from build123d import *

# Parameters (mm, degrees)
BOSS_EXTRUDE1_DEPTH = 35
SKETCH2_R           = 0.8
CUT_EXTRUDE1_DEPTH  = 6
SKETCH3_R           = 2.55
CUT_EXTRUDE2_DEPTH  = 6


with BuildPart() as part:
    # Sketch1 → Boss-Extrude1 (new body)
    with BuildSketch(Plane.XY):
        Polygon((-45.495099545, 30), (-5.495099545, 30), (-5.495099545, 0), (0, 0), (0, 35), (-51, 35), (-51, 0), (-45.495099545, 0), align=None)
    extrude(amount=-BOSS_EXTRUDE1_DEPTH)

    # Sketch2 → Cut-Extrude1 (cut)
    with BuildSketch(Plane.ZY.offset(51)):
        with Locations((-13.063320716, 15.474711623)):
            Circle(SKETCH2_R)
        with Locations((-22.063320716, 15.474711623)):
            Circle(SKETCH2_R)
    extrude(amount=-CUT_EXTRUDE1_DEPTH, mode=Mode.SUBTRACT)

    # Sketch3 → Cut-Extrude2 (cut)
    with BuildSketch(Plane(origin=(0, 35, 0), x_dir=(1, 0, 0), z_dir=(0, 1, 0))):
        with Locations(Location((-39, 31.663775096, 0), (0, 0, 180))):
            Circle(SKETCH3_R)
        with Locations(Location((-39, 11.663775096, 0), (0, 0, 180))):
            Circle(SKETCH3_R)
        with Locations(Location((-19.15, 31.663775096, 0), (0, 0, 180))):
            Circle(SKETCH3_R)
        with Locations(Location((-19.15, 11.663775096, 0), (0, 0, 180))):
            Circle(SKETCH3_R)
        with Locations(Location((-29, 21.663775096, 0), (0, 0, 180))):
            Circle(SKETCH3_R)
    extrude(amount=-CUT_EXTRUDE2_DEPTH, mode=Mode.SUBTRACT)


solid = part.part
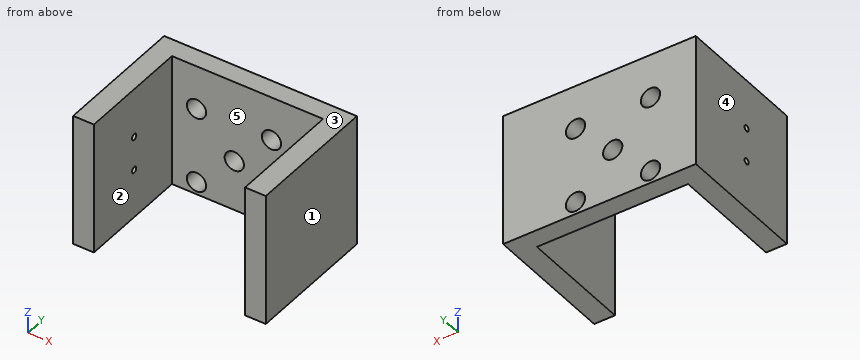
Build history of the part. All positions in model axes, mm. Face numbers are marked on the shaded views. A direction names the side the tool comes from. Round coordinates to 2 decimals unless told otherwise and drop trailing zeros. Write each loop counter-clockwise with the first axis right and the second up, starting at its lowest first coordinate (ties: lowest second). Pieces come first, ordered by that corner, then holes. Notation, with made-up numbers: M -15.75,-0.5 L 37.25,-0.5 A15 ccw 37.25,21.5 Z; hole C -15.5,-12 d10. An arc over 180 degrees is marked long. Answer in a Markdown table with one row per item.
1. Probe L1, parallel to Z at x = -19.15, y = 32.5; L2, parallel to X at y = 12, z = -12.5; L3, parallel to Y at x = -37, z = -14.5. List the from-to ranges inside material, lowest first. Write a range as [from, to].
Geometry check:
| item | result |
|---|---|
| L1 | [-35, -34.21], [-29.11, -14.21], [-9.11, 0] |
| L2 | [-51, -45.5], [-5.5, 0] |
| L3 | [30, 35] |
2. Saw through at B-B (x = -29). List the corners of the cut face in (y, z).
Geometry check:
| item | result |
|---|---|
| outline | M 30,-35 L 35,-35 L 35,-24.21 L 30,-24.21 Z; M 30,-19.11 L 35,-19.11 L 35,0 L 30,0 Z |
3. Saw through at D-D (x = -19.15). List the corners of the cut face in (y, z).
Geometry check:
| item | result |
|---|---|
| outline | M 30,-35 L 35,-35 L 35,-34.21 L 30,-34.21 Z; M 30,-29.11 L 35,-29.11 L 35,-14.21 L 30,-14.21 Z; M 30,-9.11 L 35,-9.11 L 35,0 L 30,0 Z |
4. Which spindle directions (+Z, -Z, +X, -X, +Y, -Y) get a long thin tool onto all of the face, cutting with end or side? Do the marked faces 4 and 5. Say none if no direction does.
Geometry check:
| item | result |
|---|---|
| face 4 | +Z, -Z, -X, +Y, -Y |
| face 5 | +Z, -Z, -Y |
5. Flat gauge pins, fed straight in: P1, Ø4, axis at x = -29, z = -21.66, coming from the -Y side; P2, Ø6, axis at x = -39, z = -31.66, coming from the -Y side. Where does each tip first touch, or does it go through?
Geometry check:
| item | result |
|---|---|
| P1 | through |
| P2 | y = 30 |
6. Saw through at A-A (y = 17). List the corners of the cut face in (x, z), and give its area (3 significant figures).
Geometry check:
| item | result |
|---|---|
| outline | M -51,-35 L -45.5,-35 L -45.5,0 L -51,0 Z; M -5.5,-35 L 0,-35 L 0,0 L -5.5,0 Z |
| area | 385 mm2 |
7. Mould opens along X. For the marked faces 1, 2 and 3 say: +X half, -X half, draft (parallel to the pull), parting line (faces both ways), or undercut.
Geometry check:
| item | result |
|---|---|
| face 1 | +X half |
| face 2 | undercut |
| face 3 | draft |
8. Saw through at C-C (z = -3). List the corners of the cut face in (x, y).
Geometry check:
| item | result |
|---|---|
| outline | M -51,0 L -45.5,0 L -45.5,30 L -5.5,30 L -5.5,0 L 0,0 L 0,35 L -51,35 Z |
